from build123d import *

# Parameters (mm, degrees)
SKETCH_1_W          = 170
SKETCH_1_H          = 105
EXTRUDE_1_DEPTH     = 2
SKETCH_2_R          = 1.6
SKETCH_2_R_2        = 2.1
CUT_EXTRUDE_1_DEPTH = 2


with BuildPart() as part:
    # ｽｹｯﾁ1 → ﾎﾞｽ - 押し出し1 (new body)
    with BuildSketch(Plane.XY):
        Rectangle(SKETCH_1_W, SKETCH_1_H)
    extrude(amount=EXTRUDE_1_DEPTH)

    # ｽｹｯﾁ2 → ｶｯﾄ - 押し出し1 (cut)
    with BuildSketch(Plane.XY.offset(2)):
        with Locations((0, -37.5)):
            Circle(SKETCH_2_R)
        with Locations((17, 47.5)):
            Circle(SKETCH_2_R_2)
        with Locations((-17, 47.5)):
            Circle(SKETCH_2_R_2)
    extrude(amount=-CUT_EXTRUDE_1_DEPTH, mode=Mode.SUBTRACT)


solid = part.part
The listing builds one solid part. Answer for the finished solid, in the listing's coordinates (mm). Coordinates: 2 decimals unless noted, no trailing zeros. Loops run counter-clockwise (first coordinate to the right, second up) from the corner with the lowest first, then second, coordinate; pieces in that order, holes last. Notation, with made-up numbers: (70, 53) -> (99, 53) arc R6 cw to (99, 57) -> close; hole circle Ø2 at (0.25, 13). An arc over 180 degrees is marked (long way). Answer in a Markdown table with one row per item. Add a question column.
1. The part is cut by section B-B, the plane y = 47.5. Write down the section's boundary in (x, z), then the cut area to 3 significant figures.
2. The part is cut by section A-A, the plane x = 17. Write down the section's boundary in (y, z), then the cut area to 3 significant figures.
3. The part is cut by section C-C, the plane y = -37.5. Write down the section's boundary in (x, z), then the cut area to 3 significant figures.
4. Consider line 1 (Y direction, x = 17, z = 1); line 2 (Y direction, x = 0, z = 1.2). Determine where each line is inside the solid, lowest interval first. Write a range as [from, to].
5. Determine the mould class of faces 1 (the flat face through (-1, 1, 2)), 2 (the cylindrical face through (0.74, -38.92, 1.01)) for opening direction Y: +Y half, -Y half, draft (parallel to the pull), parting line (faces both ways), or undercut.
6. A flat-ended cylindrical pin translates along its axis: P1, Ø4, axis at x = 0, y = -37.5, coming from the +Z side. Find the tip coordinate at first contact, or state that the pin passes through.
Answer below:
| question | item | result |
|---|---|---|
| 1 | outline | (-85, 0) -> (-19.1, 0) -> (-19.1, 2) -> (-85, 2) -> close; (-14.9, 0) -> (14.9, 0) -> (14.9, 2) -> (-14.9, 2) -> close; (19.1, 0) -> (85, 0) -> (85, 2) -> (19.1, 2) -> close |
| 1 | area | 323 mm2 |
| 2 | outline | (-52.5, 0) -> (45.4, 0) -> (45.4, 2) -> (-52.5, 2) -> close; (49.6, 0) -> (52.5, 0) -> (52.5, 2) -> (49.6, 2) -> close |
| 2 | area | 202 mm2 |
| 3 | outline | (-85, 0) -> (-1.6, 0) -> (-1.6, 2) -> (-85, 2) -> close; (1.6, 0) -> (85, 0) -> (85, 2) -> (1.6, 2) -> close |
| 3 | area | 334 mm2 |
| 4 | line 1 | [-52.5, 45.4], [49.6, 52.5] |
| 4 | line 2 | [-52.5, -39.1], [-35.9, 52.5] |
| 5 | face 1 | draft |
| 5 | face 2 | undercut |
| 6 | P1 | z = 2 |
